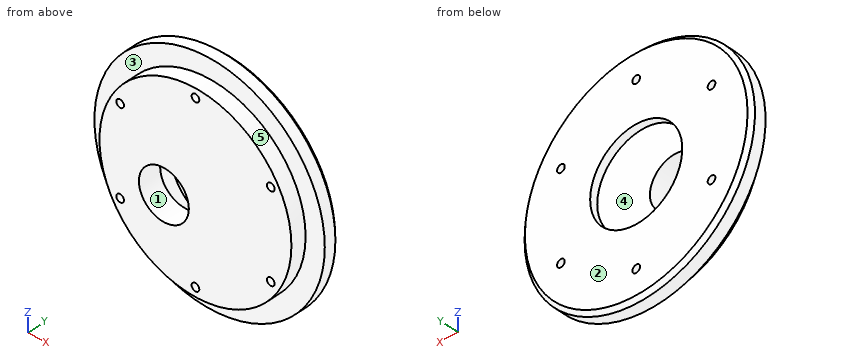
```python
from build123d import *

# Parameters (mm, degrees)
SKETCH_1_R          = 30
EXTRUDE_1_DEPTH     = 4
SKETCH_2_R          = 25
EXTRUDE_2_DEPTH     = 4
SKETCH_3_R          = 12
CUT_EXTRUDE_1_DEPTH = 2
SKETCH_4_R          = 6.5
CUT_EXTRUDE_2_DEPTH = 6
CHAMFER_1_SIZE      = 1
CUT_EXTRUDE_3_REACH = 10
SKETCH_5_R          = 1
SKETCH_6_R          = 6.5
EXTRUDE_4_DEPTH     = 6
SKETCH_9_R          = 6.5
CUT_EXTRUDE_5_DEPTH = 6


with BuildPart() as part:
    # ｽｹｯﾁ1 → ﾎﾞｽ - 押し出し1 (new body)
    with BuildSketch(Plane(origin=(0, 0, 0), x_dir=(1, 0, 0), z_dir=(0, 1, 0))):
        Circle(SKETCH_1_R)
    extrude(amount=-EXTRUDE_1_DEPTH)

    # ｽｹｯﾁ2 → ﾎﾞｽ - 押し出し2 (add)
    with BuildSketch(Plane.XZ.offset(4)):
        Circle(SKETCH_2_R)
    extrude(amount=EXTRUDE_2_DEPTH)

    # ｽｹｯﾁ3 → ｶｯﾄ - 押し出し1 (cut)
    with BuildSketch(Plane(origin=(0, 0, 0), x_dir=(1, 0, 0), z_dir=(0, 1, 0))):
        Circle(SKETCH_3_R)
    extrude(amount=-CUT_EXTRUDE_1_DEPTH, mode=Mode.SUBTRACT)

    # ｽｹｯﾁ4 → ｶｯﾄ - 押し出し2 (cut)
    with BuildSketch(Plane.XZ.offset(8)):
        with Locations((0, -14.5)):
            Circle(SKETCH_4_R)
    extrude(amount=-CUT_EXTRUDE_2_DEPTH, mode=Mode.SUBTRACT)

    # 面取り1
    chamfer_1_edges = [part.edges().sort_by_distance(p)[0] for p in [
        (-30, 0, 0),
    ]]
    chamfer(chamfer_1_edges, length=CHAMFER_1_SIZE)

    # ｽｹｯﾁ5 → ｶｯﾄ - 押し出し3 (cut, up to next)
    with BuildSketch(Plane(origin=(0, 0, 0), x_dir=(1, 0, 0), z_dir=(0, 1, 0)), mode=Mode.PRIVATE) as cut_extrude_3_sk1:
        with Locations((0, -22.65)):
            Circle(SKETCH_5_R)
    cut_extrude_3_tool1 = extrude(cut_extrude_3_sk1.sketch, amount=-CUT_EXTRUDE_3_REACH, mode=Mode.PRIVATE) & part.part
    add(cut_extrude_3_tool1.solids().sort_by_distance((0, 0, 22.65))[0], mode=Mode.SUBTRACT)
    # ｽｹｯﾁ5 → ｶｯﾄ - 押し出し3 (cut, up to next)
    with BuildSketch(Plane(origin=(0, 0, 0), x_dir=(1, 0, 0), z_dir=(0, 1, 0)), mode=Mode.PRIVATE) as cut_extrude_3_sk2:
        with Locations((-19.615475396, -11.325)):
            Circle(SKETCH_5_R)
    cut_extrude_3_tool2 = extrude(cut_extrude_3_sk2.sketch, amount=-CUT_EXTRUDE_3_REACH, mode=Mode.PRIVATE) & part.part
    add(cut_extrude_3_tool2.solids().sort_by_distance((-19.615475, 0, 11.325))[0], mode=Mode.SUBTRACT)
    # ｽｹｯﾁ5 → ｶｯﾄ - 押し出し3 (cut, up to next)
    with BuildSketch(Plane(origin=(0, 0, 0), x_dir=(1, 0, 0), z_dir=(0, 1, 0)), mode=Mode.PRIVATE) as cut_extrude_3_sk3:
        with Locations((-19.615475396, 11.325)):
            Circle(SKETCH_5_R)
    cut_extrude_3_tool3 = extrude(cut_extrude_3_sk3.sketch, amount=-CUT_EXTRUDE_3_REACH, mode=Mode.PRIVATE) & part.part
    add(cut_extrude_3_tool3.solids().sort_by_distance((-19.615475, 0, -11.325))[0], mode=Mode.SUBTRACT)
    # ｽｹｯﾁ5 → ｶｯﾄ - 押し出し3 (cut, up to next)
    with BuildSketch(Plane(origin=(0, 0, 0), x_dir=(1, 0, 0), z_dir=(0, 1, 0)), mode=Mode.PRIVATE) as cut_extrude_3_sk4:
        with Locations((0, 22.65)):
            Circle(SKETCH_5_R)
    cut_extrude_3_tool4 = extrude(cut_extrude_3_sk4.sketch, amount=-CUT_EXTRUDE_3_REACH, mode=Mode.PRIVATE) & part.part
    add(cut_extrude_3_tool4.solids().sort_by_distance((0, 0, -22.65))[0], mode=Mode.SUBTRACT)
    # ｽｹｯﾁ5 → ｶｯﾄ - 押し出し3 (cut, up to next)
    with BuildSketch(Plane(origin=(0, 0, 0), x_dir=(1, 0, 0), z_dir=(0, 1, 0)), mode=Mode.PRIVATE) as cut_extrude_3_sk5:
        with Locations((19.615475396, 11.325)):
            Circle(SKETCH_5_R)
    cut_extrude_3_tool5 = extrude(cut_extrude_3_sk5.sketch, amount=-CUT_EXTRUDE_3_REACH, mode=Mode.PRIVATE) & part.part
    add(cut_extrude_3_tool5.solids().sort_by_distance((19.615475, 0, -11.325))[0], mode=Mode.SUBTRACT)
    # ｽｹｯﾁ5 → ｶｯﾄ - 押し出し3 (cut, up to next)
    with BuildSketch(Plane(origin=(0, 0, 0), x_dir=(1, 0, 0), z_dir=(0, 1, 0)), mode=Mode.PRIVATE) as cut_extrude_3_sk6:
        with Locations((19.615475396, -11.325)):
            Circle(SKETCH_5_R)
    cut_extrude_3_tool6 = extrude(cut_extrude_3_sk6.sketch, amount=-CUT_EXTRUDE_3_REACH, mode=Mode.PRIVATE) & part.part
    add(cut_extrude_3_tool6.solids().sort_by_distance((19.615475, 0, 11.325))[0], mode=Mode.SUBTRACT)

    # ｽｹｯﾁ6 → ﾎﾞｽ - 押し出し4 (add)
    with BuildSketch(Plane.XZ.offset(8)):
        with Locations((0, -14.5)):
            Circle(SKETCH_6_R)
    extrude(amount=-EXTRUDE_4_DEPTH)

    # ｽｹｯﾁ9 → ｶｯﾄ - 押し出し5 (cut)
    with BuildSketch(Plane.XZ.offset(8)):
        with Locations((-8.227241336, -4.75)):
            Circle(SKETCH_9_R)
    extrude(amount=-CUT_EXTRUDE_5_DEPTH, mode=Mode.SUBTRACT)


solid = part.part
```
Input: part model. Units: mm. Frame: model coordinates. Face numbers are marked on the shaded views. A direction names the side the tool comes from. Coordinates: 2 decimals unless noted, no trailing zeros. Loops run counter-clockwise (first coordinate to the right, second up) from the corner with the lowest first, then second, coordinate; pieces in that order, holes last. Notation, with made-up numbers: M 53,79.5 L 87,79.5 A24 cw 87,98.5 Z; hole C -3.5,83.25 d11. An arc over 180 degrees is marked long. Answer in a Markdown table with one row per item.
1. Section A-A, the plane x = 0. Output: boundary loops of the cut face in (y, z), then the cut area to 3 significant figures.
Response:
| item | result |
|---|---|
| outline | M -8,-25 L -4,-25 L -4,-30 L -1,-30 L 0,-29 L 0,-23.65 L -8,-23.65 Z; M -8,-21.65 L 0,-21.65 L 0,-12 L -2,-12 L -2,12 L 0,12 L 0,21.65 L -8,21.65 Z; M -8,23.65 L 0,23.65 L 0,29 L -1,30 L -4,30 L -4,25 L -8,25 Z |
| area | 359 mm2 |
2. Reachability of the marked faces 1 and 2 from +Z, -Z, +X, -X, +Y, -Y: full face, straight path, thin tool, end or side. Return the list, or none.
Response:
| item | result |
|---|---|
| face 1 | -Y |
| face 2 | +Z, -Z, +X, -X, +Y |
3. Section B-B, the plane y = -5.5. Output: boundary loops of the cut face in (x, z) (3 decimals), then the cut area to 3 significant figures.
Response:
| item | result |
|---|---|
| outline | C 0,0 d50; hole C -19.615,-11.325 d2; hole C -19.615,11.325 d2; hole C -8.227,-4.75 d13; hole C 0,-22.65 d2; hole C 0,22.65 d2; hole C 19.615,-11.325 d2; hole C 19.615,11.325 d2 |
| area | 1,810 mm2 |
4. First-contact query: pin 1 (3 mm diameter, centred on y = -6, z = -8.5, fed in from +X); pin 2 (1 mm diameter, centred on x = 5, y = -1, fed in from +Z); pin 3 (3 mm diameter, centred on x = -12, z = -7, fed in from -Y); pin 4 (1.8 mm diameter, centred on x = -19.62, z = 11.32, fed in from +Y). Flat tips, straight axial feed; report the tip coordinate or a pass-through.
Response:
| item | result |
|---|---|
| pin 1 | stops at x = 24 |
| pin 2 | stops at z = 29.66 |
| pin 3 | stops at y = -2 |
| pin 4 | passes through |
5. Draft query along X for the marked faces 3, 4 and 5. Return one class per face: pulls with the +X half, pulls with the -X half, needs draft (parallel to the pull), parting line crosses it, or undercut.
Response:
| item | result |
|---|---|
| face 3 | needs draft |
| face 4 | undercut |
| face 5 | parting line crosses it |
6. Material intervals for line 1 (Z direction, x = 0, y = -4.25); line 2 (X direction, y = -2.5, z = 12); line 3 (Y direction, x = -15, z = 24), sorted ascending.
Response:
| item | result |
|---|---|
| line 1 | z = -25 to -23.65, -21.65 to 21.65, 23.65 to 25 |
| line 2 | x = -27.5 to -20.35, -18.88 to 18.88, 20.35 to 27.5 |
| line 3 | y = -4 to 0 |
